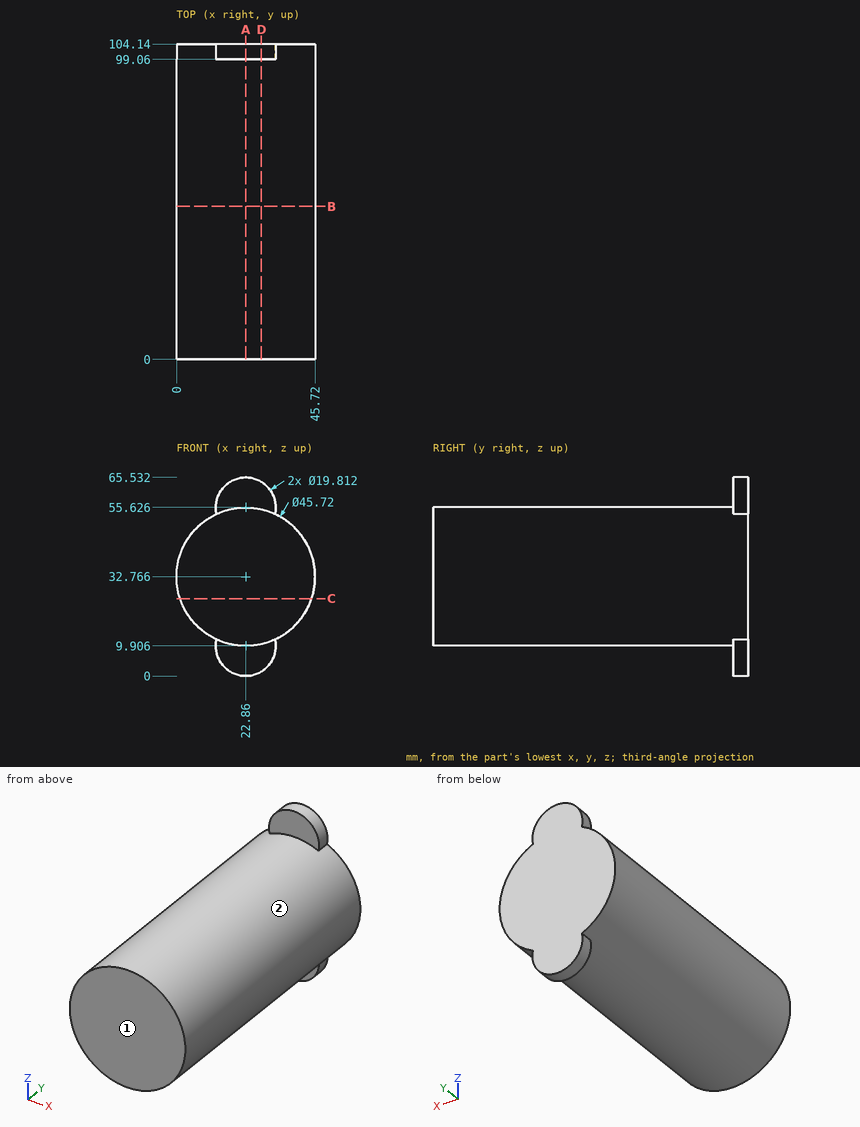
Answer from the drawing. Dimensions are ordinates in mm from the lowest x, y and z of the part. A direction names the side the tool comes from. Round coordinates to 2 decimals unless told otherwise and drop trailing zeros. Write each loop counter-clockwise with the first axis right and the second up, starting at its lowest first coordinate (ties: lowest second). Pieces come first, ordered by that corner, then holes.
1. Which of the six approach directions +Z, -Z, +X, -X, +Y, -Y give full straight-line access (tool end or side, diameter ignored) to the marked faces 1 and 2?
2. The part is cut by section A-A, the plane x = 22.86. Determine the outline of the cut face in (y, z).
3. Straight lines are drawn through the part: L1, parallel to Y at x = 26, z = 62; L2, parallel to Z at x = 32.5, y = 24; L3, parallel to Z at x = 23, y = 43. For each, find the intervals that lie inside material, in ascending order.
4. The part is cut by section B-B, the plane y = 50.5. Determine the outline of the cut face in (x, z), then the cut area to 3 significant figures.
5. The part is cut by section D-D, the plane x = 28. Determine the outline of the cut face in (y, z).
6. The part is cut by section C-C, the plane z = 25.5. Determine the outline of the cut face in (x, y), then the cut area to 3 significant figures.
7. Given pin 1 Ø10 at (y, z) = (70, 19.5) entering from +X; pin 2 Ø3 at (x, y) = (20.5, 76) entering from +Z; pin 3 Ø3 at (x, z) = (16.5, 58.5) entering from -Y; pin 4 Ø6 at (y, z) = (74.5, 34) entering from +X, each flat-ended and moving along its own axis, determine where each tip first touches the part or whether it passes through.
Values:
1. face 1: +Z, -Z, +X, -X, -Y
1. face 2: -Y
2. outline: (0, 9.91) - (99.06, 9.91) - (99.06, 0) - (104.14, 0) - (104.14, 65.53) - (99.06, 65.53) - (99.06, 55.63) - (0, 55.63) - close
3. L1: y = 99.06 to 104.14
3. L2: z = 12.04 to 53.49
3. L3: z = 9.91 to 55.63
4. outline: circle Ø45.72 at (22.86, 32.77)
4. area: 1,640 mm2
5. outline: (0, 10.49) - (99.06, 10.49) - (99.06, 1.44) - (104.14, 1.44) - (104.14, 64.09) - (99.06, 64.09) - (99.06, 55.04) - (0, 55.04) - close
6. outline: (1.19, 0) - (44.53, 0) - (44.53, 104.14) - (1.19, 104.14) - close
6. area: 4,510 mm2
7. pin 1: stops at x = 44.17
7. pin 2: stops at z = 55.61
7. pin 3: stops at y = 99.06
7. pin 4: stops at x = 45.72
